Verification items for this drawing (mm, ordinates from the low corner). A direction names the side the tool comes from. Coordinates: 2 decimals unless noted, no trailing zeros. Order: outer loops, then holes, each group sorted by start corner. A loop starts at its lowest first (then second) coordinate and runs counter-clockwise, first axis right, second up. Notation, with made-up numbers: (16, -5.5) - (55, -5.5) arc R16 cw to (55, 15.5) - close; hole circle Ø1 at (32, -36). An arc over 180 degrees is marked (long way). One line per question, with ' | ' between items. Start each with the question number.
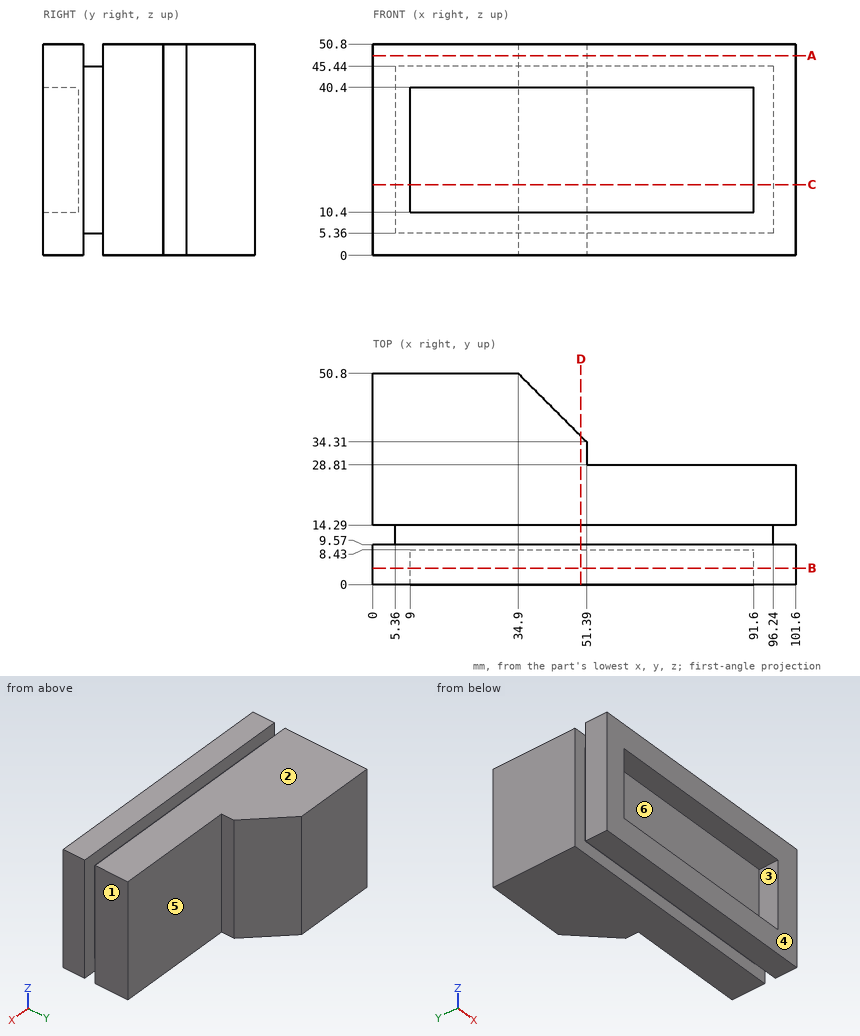
Item 1: Mould release check, pull along X, two halves, no side actions. Record for the marked faces 1, 2 and 3: +X half, -X half, draft (parallel to the pull), parting line (faces both ways), or undercut.
Item 2: Section check C-C (z = 17). Record the cut outline in (x, y).
Item 3: Section check A-A (z = 48). Record the cut outline in (x, y).
Item 4: Gauge pin test, flat ends, axial feed: pin 1 (4 mm diameter, centred on x = 82.5, y = 17, fed in from -Z); pin 2 (12 mm diameter, centred on x = 68.5, z = 31, fed in from -Y); pin 3 (15 mm diameter, centred on x = 81.5, z = 24.5, fed in from +Y); pin 4 (6 mm diameter, centred on y = 32.5, z = 19, fed in from +X). Record the tip position at first contact, or that the pin passes through.
Item 5: Thickness scan on probe 1 along Z at (x, y) = (81, 3); probe 2 along Y at (x, z) = (86, 41.5); probe 3 along X at (y, z) = (33.5, 46.5). Record the ranges inside material, lowest first. Write a range as from..to.
Item 6: Section check B-B (y = 4). Record the cut outline in (x, z), then the cut area to 3 significant figures.
Item 7: Section check D-D (x = 50). Record the cut outline in (y, z), then the cut area to 3 significant figures.
Item 8: Set-up check for the marked faces 4, 5 and 6: record each of +Z, -Z, +X, -X, +Y, -Y from which the full face is reachable in a straight line by a thin tool's end or side.
Completed:
1) face 1: +X half | face 2: draft | face 3: undercut
2) outline: (0, 0) - (9, 0) - (9, 8.43) - (91.6, 8.43) - (91.6, 0) - (101.6, 0) - (101.6, 9.57) - (96.24, 9.57) - (96.24, 14.29) - (101.6, 14.29) - (101.6, 28.81) - (51.39, 28.81) - (51.39, 34.31) - (34.9, 50.8) - (0, 50.8) - (0, 14.29) - (5.36, 14.29) - (5.36, 9.57) - (0, 9.57) - close
3) outline: (0, 0) - (101.6, 0) - (101.6, 9.57) - (0, 9.57) - close; (0, 14.29) - (101.6, 14.29) - (101.6, 28.81) - (51.39, 28.81) - (51.39, 34.31) - (34.9, 50.8) - (0, 50.8) - close
4) pin 1: stops at z = 0 | pin 2: stops at y = 8.43 | pin 3: stops at y = 28.81 | pin 4: stops at x = 51.39
5) probe 1: z = 0..10.4, 40.4..50.8 | probe 2: y = 0..28.81 | probe 3: x = 0..51.39
6) outline: (0, 0) - (101.6, 0) - (101.6, 50.8) - (0, 50.8) - close; hole (9, 10.4) - (91.6, 10.4) - (91.6, 40.4) - (9, 40.4) - close | area: 2,680 mm^2
7) outline: (0, 0) - (9.57, 0) - (9.57, 5.36) - (14.29, 5.36) - (14.29, 0) - (35.7, 0) - (35.7, 50.8) - (14.29, 50.8) - (14.29, 45.44) - (9.57, 45.44) - (9.57, 50.8) - (0, 50.8) - (0, 40.4) - (8.43, 40.4) - (8.43, 10.4) - (0, 10.4) - close | area: 1,510 mm^2
8) face 4: +Z, -Z, +X, -X, -Y | face 5: +Z, -Z, +X, +Y | face 6: -Y
